```python
from build123d import *

# Parameters (mm, degrees)
F0_R     = 1.5875
F1_DEPTH = 3.048


with BuildPart() as f1:
    # F0 (on Front) → F1 (new body)
    with BuildSketch(Plane.XZ):
        with BuildLine():
            ThreePointArc((-9.5095663313, 70.0432862662), (-6.5407566171, 63.6611249112), (0, 61.0602947442))
            ThreePointArc((0, 61.0602947442), (6.7351920908, 63.8501026534), (9.525, 70.5852947442))
            ThreePointArc((9.525, 70.5852947442), (9.5245806872, 70.6746688591), (9.5233227858, 70.7640351052))
            ThreePointArc((9.5233227858, 70.7640351052), (-0.3604400536, 80.1034725093), (-9.5095663313, 70.0432862662))
        make_face()
        with BuildLine():
            ThreePointArc((3.175, 70.5852947442), (2.2450640303, 68.3402307139), (0, 67.4102947442))
            ThreePointArc((0, 67.4102947442), (-2.2450640303, 72.8303587744), (3.175, 70.5852947442))
        make_face(mode=Mode.SUBTRACT)
        with BuildLine():
            ThreePointArc((9.525, 70.5852947442), (6.7351920908, 63.8501026534), (0, 61.0602947442))
            Line((0, 61.0602947442), (0, 56.3104947442))
            Line((0, 56.3104947442), (0, 35.6602947442))
            ThreePointArc((0, 35.6602947442), (8.3101303729, 33.311467824), (14.1611668333, 26.9600406573))
            Line((14.1611668333, 26.9600406573), (9.5233227858, 70.7640351052))
            ThreePointArc((9.5233227858, 70.7640351052), (9.5245806872, 70.6746688591), (9.525, 70.5852947442))
        make_face()
        with BuildLine():
            Line((0, 56.3104947442), (0, 61.0602947442))
            ThreePointArc((0, 61.0602947442), (-6.5407566171, 63.6611249112), (-9.5095663313, 70.0432862662))
            Line((-9.5095663313, 70.0432862662), (-13.9389716008, 27.3827084956))
            ThreePointArc((-13.9389716008, 27.3827084956), (-8.1057597329, 33.4349205322), (0, 35.6602947442))
            Line((0, 35.6602947442), (0, 56.3104947442))
        make_face()
        with Locations((-1.5875, 56.3104947442)):
            Circle(F0_R, mode=Mode.SUBTRACT)
        with BuildLine():
            ThreePointArc((14.1611668333, 26.9600406573), (8.3101303729, 33.311467824), (0, 35.6602947442))
            Line((0, 35.6602947442), (0, 22.9602947442))
            ThreePointArc((0, 22.9602947442), (2.2450640303, 22.0303587744), (3.175, 19.7852947442))
            ThreePointArc((3.175, 19.7852947442), (2.2450640303, 17.5402307139), (0, 16.6102947442))
            Line((0, 16.6102947442), (0, 3.9102947442))
            ThreePointArc((0, 3.9102947442), (8.3101303729, 6.2591216643), (14.1611668333, 12.610548831))
            ThreePointArc((14.1611668333, 12.610548831), (15.4405982475, 16.0969955751), (15.875, 19.7852947442))
            ThreePointArc((15.875, 19.7852947442), (15.4405982475, 23.4735939132), (14.1611668333, 26.9600406573))
        make_face()
        with BuildLine():
            Line((0, 22.9602947442), (0, 35.6602947442))
            ThreePointArc((0, 35.6602947442), (-8.1057597329, 33.4349205322), (-13.9389716008, 27.3827084956))
            ThreePointArc((-13.9389716008, 27.3827084956), (-15.8731151109, 20.0299203253), (-14.166468593, 12.621022792))
            ThreePointArc((-14.166468593, 12.621022792), (-8.31513102, 6.262195206), (0, 3.9102947442))
            Line((0, 3.9102947442), (0, 16.6102947442))
            ThreePointArc((0, 16.6102947442), (-3.175, 19.7852947442), (0, 22.9602947442))
        make_face()
        with BuildLine():
            ThreePointArc((0, 3.9102947442), (-8.31513102, 6.262195206), (-14.166468593, 12.621022792))
            Line((-14.166468593, 12.621022792), (-9.0839344232, -40.84978634))
            ThreePointArc((-9.0839344232, -40.84978634), (-5.6319300567, -36.0331045869), (0, -34.1897052558))
            Line((0, -34.1897052558), (0, 0))
            Line((0, 0), (0, 3.9102947442))
        make_face()
        with BuildLine():
            ThreePointArc((14.1611668333, 12.610548831), (8.3101303729, 6.2591216643), (0, 3.9102947442))
            Line((0, 3.9102947442), (0, 0))
            Line((0, 0), (0, -34.1897052558))
            ThreePointArc((0, -34.1897052558), (6.7351920908, -36.979513165), (9.525, -43.7147052558))
            Line((9.525, -43.7147052558), (36.5125, -43.7147052558))
            ThreePointArc((36.5125, -43.7147052558), (37.1472997839, -40.6043233172), (38.9501631947, -37.9914455758))
            Line((38.9501631947, -37.9914455758), (18.4799116013, -39.7163473726))
            ThreePointArc((18.4799116013, -39.7163473726), (12.1534860854, -37.3783781365), (9.8998108989, -31.0214364103))
            Line((9.8998108989, -31.0214364103), (14.1611668333, 12.610548831))
        make_face()
        with BuildLine():
            ThreePointArc((0, -34.1897052558), (-5.6319300567, -36.0331045869), (-9.0839344232, -40.84978634))
            ThreePointArc((-9.0839344232, -40.84978634), (-7.3950973803, -49.7178843915), (0.9364707331, -53.1935579061))
            ThreePointArc((0.9364707331, -53.1935579061), (7.058523526, -50.1102404667), (9.525, -43.7147052558))
            Line((9.525, -43.7147052558), (3.175, -43.7147052558))
            ThreePointArc((3.175, -43.7147052558), (-2.2450640303, -45.9597692861), (0, -40.5397052558))
            Line((0, -40.5397052558), (0, -34.1897052558))
        make_face()
        with BuildLine():
            ThreePointArc((9.525, -43.7147052558), (7.058523526, -50.1102404667), (0.9364707331, -53.1935579061))
            Line((0.9364707331, -53.1935579061), (38.9501631947, -49.4379649358))
            ThreePointArc((38.9501631947, -49.4379649358), (37.1472997839, -46.8250871944), (36.5125, -43.7147052558))
            Line((36.5125, -43.7147052558), (9.525, -43.7147052558))
        make_face()
        with BuildLine():
            ThreePointArc((36.5125, -43.7147052558), (37.1472997839, -46.8250871944), (38.9501631947, -49.4379649358))
            ThreePointArc((38.9501631947, -49.4379649358), (47.5603819386, -51.0174054719), (52.3875, -43.7147052558))
            ThreePointArc((52.3875, -43.7147052558), (47.5603819386, -36.4120050397), (38.9501631947, -37.9914455758))
            ThreePointArc((38.9501631947, -37.9914455758), (37.1472997839, -40.6043233172), (36.5125, -43.7147052558))
        make_face()
        with BuildLine():
            ThreePointArc((47.625, -43.7147052558), (44.45, -46.8897052558), (41.275, -43.7147052558))
            ThreePointArc((41.275, -43.7147052558), (44.45, -40.5397052558), (47.625, -43.7147052558))
        make_face(mode=Mode.SUBTRACT)
    extrude(amount=F1_DEPTH)


solid = f1.part
```
Design review of the part built by this model. Coordinates are the model's own, in mm. A direction names the side the tool comes from. Give positions to 0.01 mm unless a question says otherwise; leave off trailing zeros. Write each loop counter-clockwise with the first axis right and the second up, starting at its lowest first coordinate (ties: lowest second). Pieces come first, ordered by that corner, then holes.
(1) Add section A-A (x = 44.45). Give the boundary of the cut face in (y, z), and give its area (3 significant figures).
Checked values:
outline: (-3.05, -51.65) - (0, -51.65) - (0, -46.89) - (-3.05, -46.89) - close; (-3.05, -40.54) - (0, -40.54) - (0, -35.78) - (-3.05, -35.78) - close
area: 29.0 mm2
(2) Clearance check with flat-ended pins moving along their axes: pin 1 Ø1.5 at (y, z) = (-2, -36) entering from +X; pin 2 Ø1.5 at (x, y) = (6, -0.5) entering from -Z; pin 3 Ø10 at (x, z) = (41.5, -30) entering from +Y; pin 4 Ø0.9 at (x, y) = (5.5, -2) entering from +Z. State where each tip first meets the part, or that it passes through.
Checked values:
pin 1: stops at x = 48.26
pin 2: stops at z = -52.77
pin 3: passes through
pin 4: stops at z = 78.66
(3) Add section B-B (y = -1.05). Give the number of separate pieces and of enclosed holes in the cut face, and give its area (3 significant figures).
Checked values:
separate pieces: 1
enclosed holes: 5
area: 3,410 mm2
(4) Tool access review of faces 4 (the face through (12, -1.5, -9.5)), 5 (the face through (19.68, -1.5, -51.34)), 6 (the face through (6, -2, -43.715)), 7 (the face through (28.86, -1.5, -38.84)): name each direction out of +Z, -Z, +X, -X, +Y, -Y from which nothing blocks a thin tool from reaching the whole face with its end or side.
Checked values:
face 4: +X, +Y, -Y
face 5: -Z, +Y, -Y
face 6: +Y, -Y
face 7: +Z, +Y, -Y
(5) Add section C-C (z = -11.5). Give the boundary of the cut face in (x, y).
Checked values:
outline: (-11.87, -3.05) - (11.81, -3.05) - (11.81, 0) - (-11.87, 0) - close
(6) Wall thickness on line 1 along X through (y, z) = (-1.7, 21); line 2 along X through (y, z) = (-2.1, 70); line 3 along X through (y, z) = (-0.3, 9): over which ranges is each line inside the solid? List them lowest first.
Checked values:
line 1: x = -15.83 to -2.93, 2.93 to 15.83
line 2: x = -9.51 to -3.12, 3.12 to 9.6
line 3: x = -13.82 to 13.81
(7) Mouldability with a two-part tool opening along X and no side actions: class faces 1 (the face through (11.875, -1.503, 48.555)), 2 (the face through (42.74, -1.5, -41.04)), 3 (the face through (-11.66, -1.5, -13.74)) as +X half, -X half, draft (parallel to the pull), parting line (faces both ways), or undercut.
Checked values:
face 1: +X half
face 2: undercut
face 3: -X half
(8) Add section D-D (x = 25). Give the boundary of the cut face in (y, z), and give its area (3 significant figures).
Checked values:
outline: (-3.05, -50.82) - (0, -50.82) - (0, -39.17) - (-3.05, -39.17) - close
area: 35.5 mm2
